For this review, use the dimensioned drawing (mm, ordinates from the lowest corner) and the shaded views. Give positions to 0.01 mm unless a question says otherwise; leave off trailing zeros. Order: outer loops, then holes, each group sorted by start corner. A loop starts at its lowest first (then second) coordinate and runs counter-clockwise, first axis right, second up.
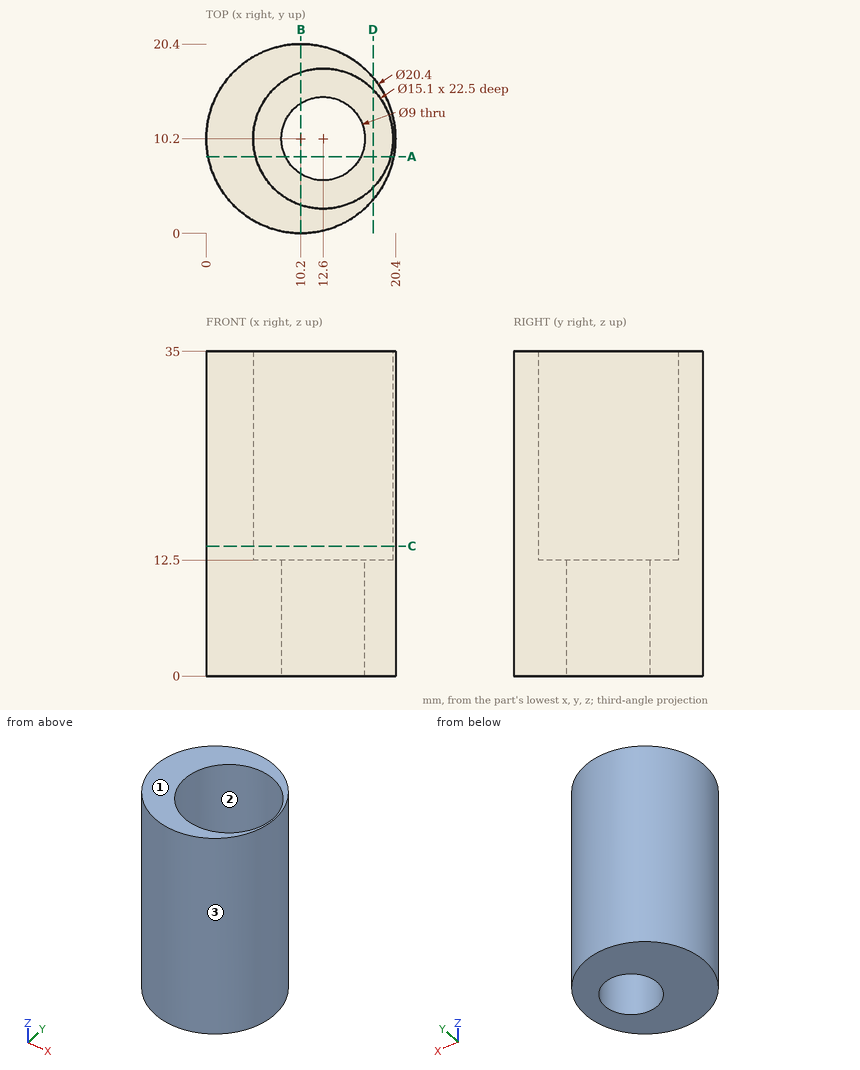
1. For pin 1 (4 mm diameter, centred on y = 6, z = 4, fed in from +X); pin 2 (10.5 mm diameter, centred on x = 12.6, y = 10.2, fed in from +Z); pin 3 (2 mm diameter, centred on y = 15.5, z = 17, fed in from +X), all flat-tipped, find the tip position at first contact; note any pin that passes through.
Recorded:
pin 1: stops at x = 20.16
pin 2: stops at z = 12.5
pin 3: stops at x = 19.45
2. Take a section at B-B (x = 10.2). State the section outline as (y, z) points.
Recorded:
outline: (0, 0) - (6.39, 0) - (6.39, 12.5) - (3.04, 12.5) - (3.04, 35) - (0, 35) - close; (14.01, 0) - (20.4, 0) - (20.4, 35) - (17.36, 35) - (17.36, 12.5) - (14.01, 12.5) - close
3. Take a section at A-A (y = 8.25). State the section outline as (x, z) points, then the cut area to 3 significant figures.
Recorded:
outline: (0.19, 0) - (8.54, 0) - (8.54, 12.5) - (5.31, 12.5) - (5.31, 35) - (0.19, 35) - close; (16.66, 0) - (20.21, 0) - (20.21, 35) - (19.89, 35) - (19.89, 12.5) - (16.66, 12.5) - close
area: 271 mm2
4. Draft analysis for pull direction X (two halves, no side actions). For the marked faces 1, 2 and 3, state which applies: pulls with the +X half, pulls with the -X half, needs draft (parallel to the pull), parting line crosses it, or undercut.
Recorded:
face 1: needs draft
face 2: undercut
face 3: parting line crosses it
5. For line 1 along X through (y, z) = (10.2, 28.75); line 2 along Z through (x, y) = (7, 12); line 3 along X through (y, z) = (10.2, 3.25), list the stretches that pass through material, from the lowest coordinate up.
Recorded:
line 1: x = 0 to 5.05, 20.15 to 20.4
line 2: z = 0 to 12.5
line 3: x = 0 to 8.1, 17.1 to 20.4
6. Take a section at C-C (z = 14). State the section outline as (x, y) points, then the cut area to 3 significant figures.
Recorded:
outline: circle Ø20.4 at (10.2, 10.2); hole circle Ø15.1 at (12.6, 10.2)
area: 148 mm2
7. Take a section at D-D (x = 18). State the section outline as (y, z) points, then the cut area to 3 significant figures.
Recorded:
outline: (3.63, 0) - (16.77, 0) - (16.77, 35) - (15.48, 35) - (15.48, 12.5) - (4.92, 12.5) - (4.92, 35) - (3.63, 35) - close
area: 223 mm2
